Geometry check sheet. Reference: the model listing, model coordinates, mm. A direction names the side the tool comes from. Coordinates: 2 decimals unless noted, no trailing zeros. Write each loop counter-clockwise with the first axis right and the second up, starting at its lowest first coordinate (ties: lowest second). Pieces come first, ordered by that corner, then holes.
from build123d import *

# Parameters (mm, degrees)
F0_W          = 43.18
F0_H          = 144.78
F1_DEPTH      = 3.81
F3_DEPTH      = 25.4
F4_T3_DEPTH   = 16.5585234346
F4_T6_DEPTH   = 16.5585234346
F4_T9_ANGLE   = 180
F4_T12_DEPTH  = 16.5585234346
F4_T15_ANGLE  = 180
F4_T18_DEPTH  = 16.5585234346
F5_R          = 1.90499
F6_R          = 0.9525
F7_DEPTH      = 1.27
F7_DEPTH_BACK = 44.45


# Not quite as in the source:
# - a fillet or chamfer that OpenCascade refuses, or shapes differently, is made with other operations: its cross-section is extruded or revolved along the edge and cut away or added
# - a fillet or chamfer is up to 0.001 mm smaller than in the source, because OpenCascade refuses the exact size


with BuildPart() as f1:
    # F0 (on Top) → F1 (new body)
    with BuildSketch(Plane.XY):
        with Locations((-6.204857491, -4.3873040367)):
            Rectangle(F0_W, F0_H)
    extrude(amount=F1_DEPTH)

    # F2 (on face) → F3 (cut)
    with BuildSketch(Plane.XY.offset(3.81)):
        with BuildLine():
            ThreePointArc((0.145142509, 57.7941725286), (-6.204857491, 64.1441725286), (-12.554857491, 57.7941725286))
            Line((-12.554857491, 57.7941725286), (0.145142509, 57.7941725286))
        make_face()
        with BuildLine():
            Line((0.145142509, 68.0026959633), (-12.554857491, 68.0026959633))
            Line((-12.554857491, 68.0026959633), (-12.554857491, 57.7941725286))
            ThreePointArc((-12.554857491, 57.7941725286), (-6.204857491, 64.1441725286), (0.145142509, 57.7941725286))
            Line((0.145142509, 57.7941725286), (0.145142509, 68.0026959633))
        make_face()
        with BuildLine():
            Line((0.145142509, 57.7941725286), (-12.554857491, 57.7941725286))
            ThreePointArc((-12.554857491, 57.7941725286), (-6.204857491, 51.4441725286), (0.145142509, 57.7941725286))
        make_face()
    extrude(amount=-F3_DEPTH, mode=Mode.SUBTRACT)

    # F4: fillet of radius 2.54 on 2 edges, made by hand


with BuildPart() as f4_tool1:
    # F4_s2 → F4_t3 (new body)
    with BuildSketch(Plane.XZ.offset(-74.3526959633)):
        with BuildLine():
            ThreePointArc((-15.094857491, 3.81), (-13.2988062667, 3.0660512242), (-12.554857491, 1.27))
            Line((-12.554857491, 1.27), (-12.554857491, 3.81))
            Line((-12.554857491, 3.81), (-15.094857491, 3.81))
        make_face()
    extrude(amount=F4_T3_DEPTH)


with BuildPart() as f4_tool4:
    # F4_s5 → F4_t6 (new body)
    with BuildSketch(Plane.XZ.offset(-74.3526959633)):
        with BuildLine():
            ThreePointArc((-15.094857491, 0), (-13.2988062667, 0.7439487758), (-12.554857491, 2.54))
            Line((-12.554857491, 2.54), (-12.554857491, 0))
            Line((-12.554857491, 0), (-15.094857491, 0))
        make_face()
    extrude(amount=F4_T6_DEPTH)


with BuildPart() as f4_tool7:
    # F4_s8 → F4_t9 (revolve)
    with BuildSketch(Plane.XZ.offset(-57.7941725286)):
        with BuildLine():
            ThreePointArc((-15.094857491, 0), (-13.2988062667, 0.7439487758), (-12.554857491, 2.54))
            Line((-12.554857491, 2.54), (-12.554857491, 0))
            Line((-12.554857491, 0), (-15.094857491, 0))
        make_face()
    revolve(axis=Axis((-6.204857491, 57.7941725286, 0), (0, 0, 1)), revolution_arc=F4_T9_ANGLE)


with BuildPart() as f4_tool10:
    # F4_s11 → F4_t12 (new body)
    with BuildSketch(Plane.XZ.offset(-57.7941725286)):
        with BuildLine():
            ThreePointArc((2.685142509, 0), (0.8890912848, 0.7439487758), (0.145142509, 2.54))
            Line((0.145142509, 2.54), (0.145142509, 0))
            Line((0.145142509, 0), (2.685142509, 0))
        make_face()
    extrude(amount=-F4_T12_DEPTH)


with BuildPart() as f4_tool13:
    # F4_s14 → F4_t15 (revolve)
    with BuildSketch(Plane.XZ.offset(-57.7941725286)):
        with BuildLine():
            ThreePointArc((-15.094857491, 3.81), (-13.2988062667, 3.0660512242), (-12.554857491, 1.27))
            Line((-12.554857491, 1.27), (-12.554857491, 3.81))
            Line((-12.554857491, 3.81), (-15.094857491, 3.81))
        make_face()
    revolve(axis=Axis((-6.204857491, 57.7941725286, 3.81), (0, 0, 1)), revolution_arc=F4_T15_ANGLE)


with BuildPart() as f4_tool16:
    # F4_s17 → F4_t18 (new body)
    with BuildSketch(Plane.XZ.offset(-57.7941725286)):
        with BuildLine():
            ThreePointArc((2.685142509, 3.81), (0.8890912848, 3.0660512242), (0.145142509, 1.27))
            Line((0.145142509, 1.27), (0.145142509, 3.81))
            Line((0.145142509, 3.81), (2.685142509, 3.81))
        make_face()
    extrude(amount=-F4_T18_DEPTH)


with BuildPart() as f1_1:
    add(f1.part)

    # F4_t19: cut F4_tool1, F4_tool4, F4_tool7, F4_tool10, F4_tool13, F4_tool16
    add([f4_tool1.part, f4_tool4.part, f4_tool7.part, f4_tool10.part, f4_tool13.part, f4_tool16.part], mode=Mode.SUBTRACT)

    # F5 (radius 1.905 in the source; OpenCascade refuses exactly that, so slightly less here)
    f5_edges = [f1_1.edges().sort_by_distance(p)[0] for p in [
        (-6.204857, -76.777304, 3.81),
        (-6.204857, -76.777304, 0),
    ]]
    fillet(f5_edges, radius=F5_R)

    # F6 (on face) → F7 (join, two sides)
    with BuildSketch(Plane(origin=(-27.794857491, 0, 0), x_dir=(0, -1, 0), z_dir=(-1, 0, 0))) as f7_sk:
        with Locations((74.8723040367, 1.905)):
            Circle(F6_R)
    extrude(amount=F7_DEPTH)
    extrude(f7_sk.sketch, amount=-F7_DEPTH_BACK)


solid = f1_1.part
1. Access from +Z, -Z, +X, -X, +Y, -Y to the whole of each face (thin tool, end or side, straight path). Record for faces 1 (the cylindrical face through (-13.558, 62.97, 0.518)), 2 (the flat face through (-7, -2, 0)), 3 (the cylindrical face through (-13.558, 62.97, 3.292)).
Computed values:
face 1: -Z, +Y
face 2: -Z, +X, -X, +Y, -Y
face 3: +Z, +Y
2. Thickness scan on line 1 along X through (y, z) = (3.5, 2.4); line 2 along Y through (x, z) = (6, 1.7); line 3 along X through (y, z) = (52, 3). Record the ranges inside material, lowest first.
Computed values:
line 1: x = -27.79 to 15.39
line 2: y = -76.77 to 68
line 3: x = -27.79 to -10.19, -2.22 to 15.39
3. Draft check along X on faces 4 (the cylindrical face through (1.148, 62.827, 0.518)), 5 (the cylindrical face through (1.148, 62.827, 3.292)), 6 (the flat face through (15.385, -5, 2)), 7 (the flat face through (-7, -2, 3.81)). Enter one of: released by +X, released by -X, zero draft, split by the parting line, or undercut.
Computed values:
face 4: undercut
face 5: undercut
face 6: released by +X
face 7: zero draft
4. Gauge pin test, flat end, axial feed: pin 1 Ø1.9 at (y, z) = (-13.5, 1) entering from +X. Record the tip position at first contact, or that the pin passes through.
Computed values:
pin 1: stops at x = 15.39
5. Sectioned sample at A-A, the plane y = -3. Record the boundary of the cut face in (x, z).
Computed values:
outline: (-27.79, 0) - (15.39, 0) - (15.39, 3.81) - (-27.79, 3.81) - close
